```python
from build123d import *

# Parameters (mm, degrees)
SKETCH1_W           = 60
SKETCH1_H           = 90
BOSS_EXTRUDE1_DEPTH = 15
SKETCH2_R           = 30
BOSS_EXTRUDE2_DEPTH = 25
SKETCH3_R           = 8
BOSS_EXTRUDE3_DEPTH = 15


with BuildPart() as part:
    # Sketch1 → Boss-Extrude1 (new body)
    with BuildSketch(Plane.XY):
        Rectangle(SKETCH1_W, SKETCH1_H)
    extrude(amount=BOSS_EXTRUDE1_DEPTH)

    # Sketch2 → Boss-Extrude2 (add)
    with BuildSketch(Plane.XY.offset(15)):
        Circle(SKETCH2_R)
        with BuildLine():
            Line((-4, -14.456832295), (-4, -18))
            Line((-4, -18), (4, -18))
            Line((4, -18), (4, -14.456832295))
            ThreePointArc((4, -14.456832295), (0, 15), (-4, -14.456832295))
        make_face(mode=Mode.SUBTRACT)
    extrude(amount=BOSS_EXTRUDE2_DEPTH)

    # Sketch3 → Boss-Extrude3 (add)
    with BuildSketch(Plane(origin=(0, 45, 0), x_dir=(1, 0, 0), z_dir=(0, 1, 0))):
        with BuildLine():
            Line((30, 0), (22.03289839, 26.599347585))
            ThreePointArc((22.03289839, 26.599347585), (0, 43), (-22.03289839, 26.599347585))
            Line((-22.03289839, 26.599347585), (-30, 0))
            Line((-30, 0), (30, 0))
        make_face()
        with Locations(Location((0, 20, 0), (0, 0, 180))):
            Circle(SKETCH3_R, mode=Mode.SUBTRACT)
    boss_extrude3 = extrude(amount=-BOSS_EXTRUDE3_DEPTH)

    # Mirror1: Boss-Extrude3 across plane
    add(boss_extrude3.mirror(Plane.ZX))


solid = part.part
```
Work out the finished part from the listing and answer in its coordinate system (mm). A direction names the side the tool comes from. Coordinates: 2 decimals unless noted, no trailing zeros. Loops run counter-clockwise (first coordinate to the right, second up) from the corner with the lowest first, then second, coordinate; pieces in that order, holes last.
1) For faces 4 (the flat face through (6, 30, -12)), 5 (the flat face through (0, -32, 15)), 6 (the flat face through (0, -18, 27)), 7 (the flat face through (0, 33, 15)), determine the directions among +Z, -Z, +X, -X, +Y, -Y from which every point of the face is accessible in a straight line to the end or side of a thin tool.
Results:
face 4: -Z, +X, -X
face 5: +Z, -Y
face 6: +Z
face 7: +Z, +Y
2) Flat-ended cylindrical pins translate along their axes: pin 1 (12 mm diameter, centred on x = 0.5, y = -20.5, fed in from -Z); pin 2 (2.5 mm diameter, centred on x = 0.5, z = 31, fed in from +Y); pin 3 (1.1 mm diameter, centred on y = -16, z = 21.5, fed in from +X); pin 4 (18.5 mm diameter, centred on x = 0, z = -20, fed in from +Y). Find the tip coordinate at first contact, or state that the pin passes through.
Results:
pin 1: stops at z = 0
pin 2: stops at y = 30
pin 3: stops at x = 25.72
pin 4: stops at y = 45
3) Section D-D (z = -20) is taken. Give the vertices of the cut face in (x, y).
Results:
outline: (-24.01, -45) - (-8, -45) - (-8, -30) - (-24.01, -30) - close; (-24.01, 30) - (-8, 30) - (-8, 45) - (-24.01, 45) - close; (8, -45) - (24.01, -45) - (24.01, -30) - (8, -30) - close; (8, 30) - (24.01, 30) - (24.01, 45) - (8, 45) - close
4) Section B-B (y = 32.5) is taken. Give the vertices of the cut face in (x, z).
Results:
outline: (-30, 0) - (-22.03, -26.6) arc R23 ccw to (22.03, -26.6) - (30, 0) - (30, 15) - (-30, 15) - close; hole circle Ø16 at (0, -20)
5) Consider probe 1 along Y at (x, z) = (-3.5, -1.5); probe 2 along X at (y, z) = (13, 31.5); probe 3 along Z at (x, y) = (-12, 19). Determine where each line is inside the solid, lowest interval first.
Results:
probe 1: y = -45 to -30, 30 to 45
probe 2: x = -27.04 to -7.48, 7.48 to 27.04
probe 3: z = 0 to 40
6) Section A-A (x = 0) is taken. Give the vertices of the cut face in (y, z).
Results:
outline: (-45, -43) - (-30, -43) - (-30, -28) - (-45, -28) - close; (-45, -12) - (-30, -12) - (-30, 0) - (30, 0) - (30, -12) - (45, -12) - (45, 15) - (30, 15) - (30, 40) - (15, 40) - (15, 15) - (-18, 15) - (-18, 40) - (-30, 40) - (-30, 15) - (-45, 15) - close; (30, -43) - (45, -43) - (45, -28) - (30, -28) - close
7) For a pull along X with two mould halves and no side action, classify faces 1 (the flat face through (0, -1, 15)), 2 (the cylindrical face through (0, 38, -43)), 3 (the flat face through (6, -30, -12)) as +X half, -X half, draft (parallel to the pull), parting line (faces both ways), or undercut.
Results:
face 1: undercut
face 2: parting line
face 3: draft
8) Section C-C (z = 21.5) is taken. Give the vertices of the cut face in (x, y).
Results:
outline: circle Ø60 at (0, 0); hole (-4, -18) - (4, -18) - (4, -14.46) arc R15 ccw (long way) to (-4, -14.46) - close
